Geometry check sheet. Reference: the model listing, model coordinates, mm. Round coordinates to 2 decimals unless told otherwise and drop trailing zeros. Order: outer loops, then holes, each group sorted by start corner. A loop starts at its lowest first (then second) coordinate and runs counter-clockwise, first axis right, second up. Notation, with made-up numbers: (38.5, -8) - (68.5, -8) arc R10 ccw to (68.5, 9) - close; hole circle Ø4 at (47.5, 52). An arc over 180 degrees is marked (long way). Use a Markdown table: item, result. Add a question column.
(1) Section check B-B on y = 0.7. Record the boundary of the cut face in (x, z).
(2) Section check A-A on x = 9. Record the boundary of the cut face in (y, z), then the cut area to 3 significant figures.
(3) Section check D-D on x = 2.75. Record the boundary of the cut face in (y, z).
(4) Section check C-C on z = 0.5. Record the boundary of the cut face in (x, y).
(5) Thickness scan on line 1 along Z through (x, y) = (9.5, 1.4); line 2 along Z through (x, y) = (14.25, 0.8); line 3 along X through (y, z) = (1.4, 0.5). Record the ranges inside material, lowest first. Write a range as [from, to].
(6) Gauge pin test, flat ends, axial feed: P1, Ø1.1, axis at x = 0.5, y = 1.5, coming from the +Z side; P2, Ø0.6, axis at y = 1, z = -36, coming from the -X side; P3, Ø0.8, axis at y = 1, z = -34.5, coming from the +X side. Record the tip position at first contact, or that the pin passes through.
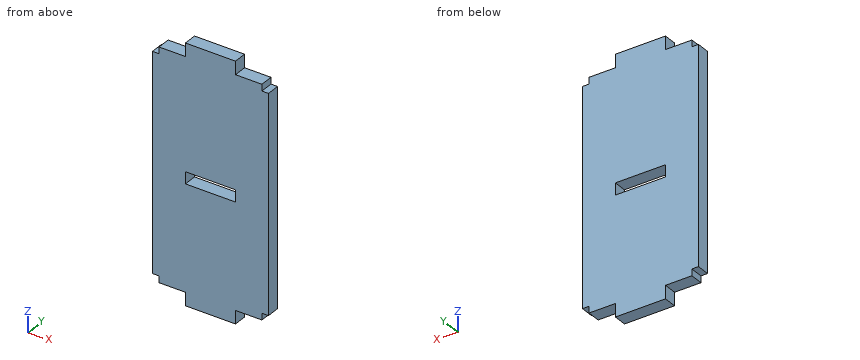
```python
from build123d import *

# Parameters (mm, degrees)
SKETCH_1_W      = 7.6
SKETCH_1_H      = 1.8
EXTRUDE_1_DEPTH = 2


with BuildPart() as part:
    # 草图1 → 凸台-拉伸1 (new body)
    with BuildSketch(Plane(origin=(0, 0, 0), x_dir=(1, 0, 0), z_dir=(0, 1, 0))):
        Polygon((1, 1), (1, 0), (5, 0), (5, -2), (12.6, -2), (12.6, 0), (16.6, 0), (16.6, 1), (17.6, 1), (17.6, 33.8), (16.6, 33.8), (16.6, 34.8), (12.6, 34.8), (12.6, 36.8), (5, 36.8), (5, 34.8), (1, 34.8), (1, 33.8), (0, 33.8), (0, 1), align=None)
        with Locations((8.8, 17.9)):
            Rectangle(SKETCH_1_W, SKETCH_1_H, mode=Mode.SUBTRACT)
    extrude(amount=EXTRUDE_1_DEPTH)


solid = part.part
```
Check sheet entries:
| question | item | result |
|---|---|---|
| 1 | outline | (0, -33.8) - (1, -33.8) - (1, -34.8) - (5, -34.8) - (5, -36.8) - (12.6, -36.8) - (12.6, -34.8) - (16.6, -34.8) - (16.6, -33.8) - (17.6, -33.8) - (17.6, -1) - (16.6, -1) - (16.6, 0) - (12.6, 0) - (12.6, 2) - (5, 2) - (5, 0) - (1, 0) - (1, -1) - (0, -1) - close; hole (5, -18.8) - (12.6, -18.8) - (12.6, -17) - (5, -17) - close |
| 2 | outline | (0, -36.8) - (2, -36.8) - (2, -18.8) - (0, -18.8) - close; (0, -17) - (2, -17) - (2, 2) - (0, 2) - close |
| 2 | area | 74.0 mm2 |
| 3 | outline | (0, -34.8) - (2, -34.8) - (2, 0) - (0, 0) - close |
| 4 | outline | (5, 0) - (12.6, 0) - (12.6, 2) - (5, 2) - close |
| 5 | line 1 | z = [-36.8, -18.8], [-17, 2] |
| 5 | line 2 | z = [-34.8, 0] |
| 5 | line 3 | x = [5, 12.6] |
| 6 | P1 | stops at z = 0 |
| 6 | P2 | stops at x = 5 |
| 6 | P3 | stops at x = 16.6 |
